Solid Edge part; units mm, degrees
sketch "Sketch1" plane through (0, 0, 0) normal (0, -1, 0) x (1, 0, 0)
  line L0 (10, -10) -> (10, 10)
  line L1 (10, 10) -> (-10, 10)
  line L2 (-10, 10) -> (-10, -10)
  line L3 (-10, -10) -> (10, -10)
  circle A0 centre (0, 0) radius 2.1
extrude "Protrusion1" add sketch "Sketch1" along normal mid plane 158
sketch "Sketch2" plane through (0, 0, 0) normal (0, -1, 0) x (1, 0, 0)
  line L0 (5.5, 6.56) -> (2.84, 3.9)
  line L1 (2.84, 3.9) -> (-2.84, 3.9)
  line L2 (-5.5, 6.56) -> (-2.84, 3.9)
  line L3 (-5.5, 8.2) -> (-5.5, 6.56)
  line L4 (-3.125, 8.2) -> (-5.5, 8.2)
  line L5 (-3.125, 10) -> (-3.125, 8.2)
  line L6 (-3.125, 10) -> (3.125, 10)
  line L7 (3.125, 10) -> (3.125, 8.2)
  line L8 (3.125, 8.2) -> (5.5, 8.2)
  line L9 (5.5, 8.2) -> (5.5, 6.56)
extrude "Cutout1" cut sketch "Sketch2" along normal through all and the other way through all
chamfer "Chaflán_1" distance 1.5 angle 45 2 edges at (-3.125, 0, 10) (3.125, 0, 10)
pattern_circular "Pattern1" count 4 over 360 about axis through (0, -79, 0) along (0, 1, 0) of "Cutout1", "Chaflán_1"
fillet "Redondeo_3" radius 0.5 4 edges at (-10, 0, 10) (10, 0, 10) (10, 0, -10) (-10, 0, -10)
The model under review builds one solid part; all positions refer to its coordinate system, in mm. A direction names the side the tool comes from. Round coordinates to 2 decimals unless told otherwise and drop trailing zeros. Write each loop counter-clockwise with the first axis right and the second up, starting at its lowest first coordinate (ties: lowest second). Pieces come first, ordered by that corner, then holes. Notation, with made-up numbers: M 1,-27 L 47,-27 A21 cw 47,-22 Z; hole C -10.75,-15 d11. An arc over 180 degrees is marked long. Answer as CSV lines item,"result". Start each with the question number.
Q1. Tool access review of faces 1 (the face through (-10, 1, 7)), 2 (the face through (-3.9, 1, 0)), 3 (the face through (10, 1, -7)), 4 (the face through (3.9, 1, 0)), 5 (the face through (5.25, 1.11, -4.19)): name each direction out of +Z, -Z, +X, -X, +Y, -Y from which nothing blocks a thin tool from reaching the whole face with its end or side.
Q2. Clearance check with flat-ended pins moving along their axes: P1, Ø2, axis at y = -54, z = -2.5, coming from the +X side (3 decimals); P2, Ø3, axis at x = -1, y = 16.5, coming from the -Z side; P3, Ø6, axis at y = 7.5, z = 1, coming from the +X side (3 decimals). State where each tip first meets the part, or that it passes through.
Q3. Consider section A-A, the plane x = 0. Give the boundary of the cut face in (y, z).
Q4. The part is to be moulded in two halves that separate along Z. For faces 6 (the face through (5.25, 1.11, 4.19)), 7 (the face through (-5.25, 1.11, -4.19)), 8 (the face through (-7, 1, -10)), 9 (the face through (0, 1, 3.9)), say which applies: +Z half, -Z half, draft (parallel to the pull), parting line (faces both ways), or undercut.
Q5. Wall thickness on line 1 along Z through (x, y) = (0, 28); line 2 along Z through (x, y) = (-8.5, -44) (3 decimals); line 3 along Z through (x, y) = (5.25, -67.5): over which ranges is each line inside the solid? List them lowest first.
Q6. Consider section B-B, the plane z = 0. Give the boundary of the cut face in (x, y).
Result set:
1,face 1,"+Z, -Z, -X, +Y, -Y"
1,face 2,"-X, +Y, -Y"
1,face 3,"+Z, -Z, +X, +Y, -Y"
1,face 4,"+X, +Y, -Y"
1,face 5,"+Y, -Y"
2,P1,"stops at x = 8.875"
2,P2,"stops at z = -3.9"
2,P3,"stops at x = 9.375"
3,outline,"M -79,-3.9 L 79,-3.9 L 79,-2.1 L -79,-2.1 Z; M -79,2.1 L 79,2.1 L 79,3.9 L -79,3.9 Z"
4,face 6,"undercut"
4,face 7,"undercut"
4,face 8,"-Z half"
4,face 9,"+Z half"
5,line 1,"z = -3.9 to -2.1, 2.1 to 3.9"
5,line 2,"z = -10 to -3.125, 3.125 to 10"
5,line 3,"z = -10 to -8.2, -6.31 to -4.19, 4.19 to 6.31, 8.2 to 10"
6,outline,"M -3.9,-79 L -2.1,-79 L -2.1,79 L -3.9,79 Z; M 2.1,-79 L 3.9,-79 L 3.9,79 L 2.1,79 Z"
